```python
from build123d import *

# Parameters (mm, degrees)
CUT_EXTRUDE7_DEPTH = 4.35
CUT_EXTRUDE8_DEPTH = 63.5


with BuildPart() as part:
    # Sketch1 → Revolve1 (revolve)
    with BuildSketch(Plane(origin=(0, 0, 0), x_dir=(0, 0, -1), z_dir=(1, 0, 0))):
        with BuildLine():
            Line((0, 0), (0, 23.4))
            ThreePointArc((0, 23.4), (-0.585786438, 24.814213562), (-2, 25.4))
            Line((-2, 25.4), (-354, 25.4))
            ThreePointArc((-354, 25.4), (-355.414213562, 24.814213562), (-356, 23.4))
            Line((-356, 23.4), (-356, 0))
            Line((-356, 0), (0, 0))
        make_face()
    revolve(axis=Axis((0, 0, 0), (0, 0, 1)))

    # Sketch6 → Cut-Extrude7 (cut)
    with BuildSketch(Plane(origin=(25.4, 0, 0), x_dir=(0, 0, -1), z_dir=(1, 0, 0))):
        with BuildLine():
            Line((0, 6.35), (-43.65, 6.35))
            ThreePointArc((-43.65, 6.35), (-50, 0), (-43.65, -6.35))
            Line((-43.65, -6.35), (0, -6.35))
            Line((0, -6.35), (0, 6.35))
        make_face()
    extrude(amount=-CUT_EXTRUDE7_DEPTH, mode=Mode.SUBTRACT)

    # Sketch7 → Cut-Extrude8 (cut)
    with BuildSketch(Plane.XY.offset(247.75)):
        with BuildLine():
            Line((-5, 24.903011866), (-5, 14.903011866))
            Line((-5, 14.903011866), (5, 14.903011866))
            Line((5, 14.903011866), (5, 24.903011866))
            ThreePointArc((5, 24.903011866), (0, 25.4), (-5, 24.903011866))
        make_face()
    extrude(amount=-CUT_EXTRUDE8_DEPTH, mode=Mode.SUBTRACT)


solid = part.part
```
Verification items for the finished model (mm, model axes). A direction names the side the tool comes from. Round coordinates to 2 decimals unless told otherwise and drop trailing zeros. Write each loop counter-clockwise with the first axis right and the second up, starting at its lowest first coordinate (ties: lowest second). Pieces come first, ordered by that corner, then holes.
1. Draft check along X on faces 4 (the flat face through (21.05, 0, 25)), 5 (the flat face through (0, 0, 356)), 6 (the flat face through (0, 20, 247.75)), 7 (the flat face through (0, 14.903, 216)). Enter one of: +X half, -X half, draft (parallel to the pull), parting line (faces both ways), or undercut.
2. Gauge pin test, flat ends, axial feed: P1, Ø2, axis at x = -15.5, z = 38.5, coming from the +Y side; P2, Ø3, axis at y = -18, z = 58, coming from the -X side; P3, Ø8, axis at y = -7, z = 164, coming from the +X side. Record the tip position at first contact, or that the pin passes through.
3. Scan lines: L1, parallel to Y at x = -12.5, z = 108; L2, parallel to Y at x = -4.5, z = 211. Record each from-to range of solid material in increasing order.
4. Section check B-B on z = 317. Enter the section's corners in (x, y).
5. Section check A-A on x = 0. Enter the section's corners in (y, z), plus the area to 3 significant figures.
6. Access from +Z, -Z, +X, -X, +Y, -Y to the whole of each face (thin tool, end or side, straight path). Record for faces 1 (the flat face through (-1, 0, 0)), 2 (the flat face through (0, 20, 184.25)), 3 (the cylindrical face through (23, 0, 50)).
Answer:
1. face 4: +X half
1. face 5: draft
1. face 6: undercut
1. face 7: undercut
2. P1: stops at y = 20.85
2. P2: stops at x = -19.31
2. P3: stops at x = 25.22
3. L1: y = -22.11 to 22.11
3. L2: y = -25 to 14.9
4. outline: circle Ø50.8 at (0, 0)
5. outline: (-25.4, 2) arc R2 ccw to (-23.4, 0) - (23.4, 0) arc R2 ccw to (25.4, 2) - (25.4, 184.25) - (14.9, 184.25) - (14.9, 247.75) - (25.4, 247.75) - (25.4, 354) arc R2 ccw to (23.4, 356) - (-23.4, 356) arc R2 ccw to (-25.4, 354) - close
5. area: 17,400 mm2
6. face 1: -Z, +X, -X, +Y, -Y
6. face 2: +Y
6. face 3: -Z, +X
